```python
from build123d import *

# Parameters (mm, degrees)
SKETCH1_R                         = 12.7
BOSS_EXTRUDE1_DEPTH               = 177.8
F_1_2_13_TAPPED_HOLE1_D           = 10.71626
F_1_2_13_TAPPED_HOLE1_DEPTH       = 25.4
F_1_2_13_TAPPED_HOLE1_CSINK_D     = 13.97
F_1_2_13_TAPPED_HOLE1_CSINK_ANGLE = 100
F_1_2_13_TAPPED_HOLE1_TIP         = 3.219489309
F_3_8_16_TAPPED_HOLE1_D           = 7.9375
F_3_8_16_TAPPED_HOLE1_DEPTH       = 25.4
F_3_8_16_TAPPED_HOLE1_CSINK_D     = 10.795
F_3_8_16_TAPPED_HOLE1_CSINK_ANGLE = 100
F_3_8_16_TAPPED_HOLE1_TIP         = 2.384665582


with BuildPart() as part:
    # Sketch1 → Boss-Extrude1 (new body)
    with BuildSketch(Plane(origin=(0, 0, 0), x_dir=(1, 0, 0), z_dir=(0, 1, 0))):
        with Locations(Location((0, 0, 0), (0, 0, 270))):
            Circle(SKETCH1_R)
    extrude(amount=BOSS_EXTRUDE1_DEPTH)

    # 1/2-13 Tapped Hole1
    with Locations(Plane(origin=(0, 0, 0), x_dir=(-1, 0, 0), z_dir=(0, -1, 0))):
        with Locations((0, 0)):
            CounterSinkHole(F_1_2_13_TAPPED_HOLE1_D / 2, F_1_2_13_TAPPED_HOLE1_CSINK_D / 2, depth=F_1_2_13_TAPPED_HOLE1_DEPTH, counter_sink_angle=F_1_2_13_TAPPED_HOLE1_CSINK_ANGLE)
            with Locations((0, 0, -(F_1_2_13_TAPPED_HOLE1_DEPTH + F_1_2_13_TAPPED_HOLE1_TIP / 2))):  # 118° drill point
                Cone(0, F_1_2_13_TAPPED_HOLE1_D / 2, F_1_2_13_TAPPED_HOLE1_TIP, mode=Mode.SUBTRACT)

    # 3/8-16 Tapped Hole1
    with Locations(Plane(origin=(0, 177.8, 0), x_dir=(1, 0, 0), z_dir=(0, 1, 0))):
        with Locations((0, 0)):
            CounterSinkHole(F_3_8_16_TAPPED_HOLE1_D / 2, F_3_8_16_TAPPED_HOLE1_CSINK_D / 2, depth=F_3_8_16_TAPPED_HOLE1_DEPTH, counter_sink_angle=F_3_8_16_TAPPED_HOLE1_CSINK_ANGLE)
            with Locations((0, 0, -(F_3_8_16_TAPPED_HOLE1_DEPTH + F_3_8_16_TAPPED_HOLE1_TIP / 2))):  # 118° drill point
                Cone(0, F_3_8_16_TAPPED_HOLE1_D / 2, F_3_8_16_TAPPED_HOLE1_TIP, mode=Mode.SUBTRACT)


solid = part.part
```
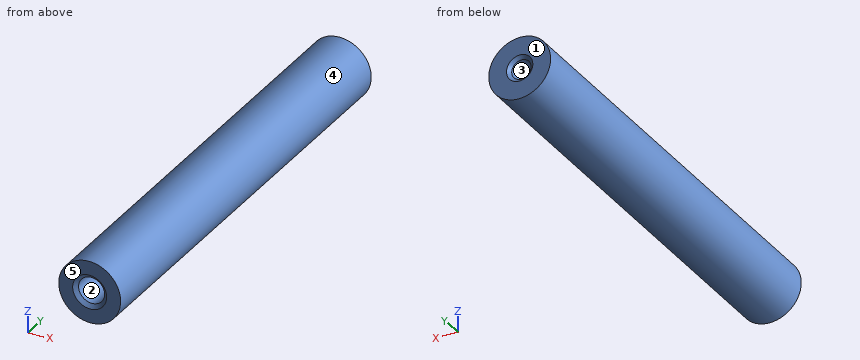
The model under review builds one solid part; all positions refer to its coordinate system, in mm. Face numbers are marked on the shaded views. A direction names the side the tool comes from. Round coordinates to 2 decimals unless told otherwise and drop trailing zeros. Order: outer loops, then holes, each group sorted by start corner. A loop starts at its lowest first (then second) coordinate and runs counter-clockwise, first axis right, second up. Notation, with made-up numbers: (-40, 89) -> (-16, 89) arc R33 ccw to (-16, 120) -> close; hole circle Ø5 at (-12, -8). An arc over 180 degrees is marked (long way). One line per item, written item: value. Start each with the question number.
Q1. Take a section at C-C (x = 9). Write out the cut boundary in (y, z).
Q2. Take a section at B-B (y = 161). Write out the cut boundary in (x, z).
Q3. Mouldability with a two-part tool opening along X and no side actions: class the marked faces 3, 4 and 5 as released by +X, released by -X, zero draft, split by the parting line, or undercut.
Q4. Clearance check with flat-ended pins moving along their axes: pin 1 Ø2 at (y, z) = (144, -1.5) entering from -X; pin 2 Ø10.5 at (x, z) = (0, 0) entering from +Y; pin 3 Ø2 at (y, z) = (129.5, -4) entering from +X. State where each tip first meets the part, or that it passes through.
Q5. Wall thickness on line 1 (X direction, y = 158.5, z = 11.5); line 2 (X direction, y = 20, z = -3.25): over which ranges is each line inside the solid? List them lowest first.
Q6. Machinability: for the marked faces 1 and 2, which of the approach directions +Z, -Z, +X, -X, +Y, -Y give a long, thin tool a straight path to every point of the face, cutting with its end or side? Answer none if there is none.
Q7. Take a section at A-A (y = 45.5). Write out the cut boundary in (x, z), and give its area (3 significant figures).
Reported:
1. outline: (0, -8.96) -> (177.8, -8.96) -> (177.8, 8.96) -> (0, 8.96) -> close
2. outline: circle Ø25.4 at (0, 0); hole circle Ø7.94 at (0, 0)
3. face 3: undercut
3. face 4: split by the parting line
3. face 5: zero draft
4. pin 1: stops at x = -12.69
4. pin 2: stops at y = 177.68
4. pin 3: stops at x = 12.34
5. line 1: x = -5.39 to 5.39
5. line 2: x = -12.28 to -4.26, 4.26 to 12.28
6. face 1: +Z, -Z, +X, -X, +Y
6. face 2: -Y
7. outline: circle Ø25.4 at (0, 0)
7. area: 507 mm2
